Job drawing, mm, ordinate dimensions from the low corner. One solid piece. Give positions to 0.01 mm unless a question says otherwise; leave off trailing zeros. Write each loop counter-clockwise with the first axis right and the second up, starting at its lowest first coordinate (ties: lowest second). Pieces come first, ordered by that corner, then holes. Notation, with made-up numbers: M 57.25,63.25 L 115.25,63.25 A22 cw 115.25,83.25 Z; hole C 38,25 d6. An arc over 180 degrees is marked long. Use CSV: the item, a comma, the result in double quotes. Start each with the question number.
Item 1: Cut at D-D (y = 9.75). List the corners of the cut face in (x, z), then the cut area to 3 significant figures.
Item 2: Cut at C-C (x = 6.25). List the corners of the cut face in (y, z).
Item 3: Cut at A-A (x = 18.05). List the corners of the cut face in (y, z) (3 decimals).
Item 4: Pin check, flat tip, straight feed: pin 1 (2 mm diameter, centred on x = 17, z = 7.5, fed in from -Y). Stop position of the tip, or through.
Item 5: Cut at B-B (y = 2.79). List the corners of the cut face in (x, z) (3 decimals).
Item 6: Drill centre line: line 1 (Z direction, x = 7.25, y = 7.25). Where is it in solid material? Low to high. Write a range as [from, to].
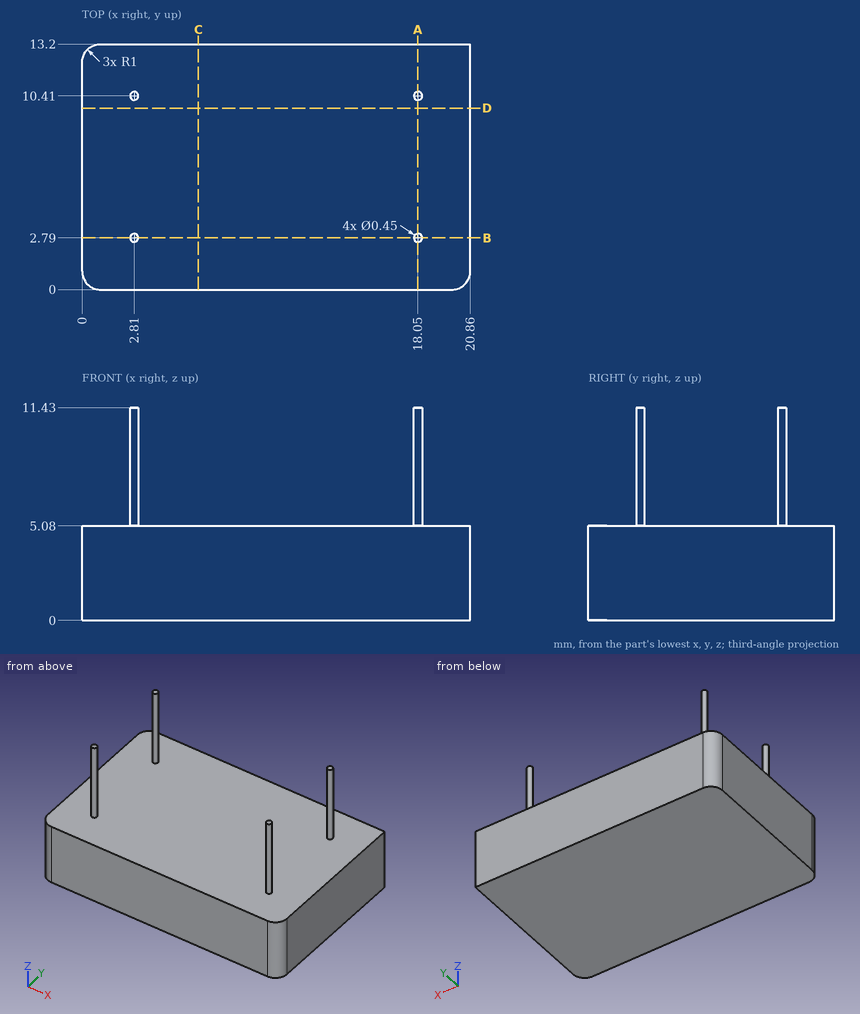
Worked answers:
1,outline,"M 0,0 L 20.86,0 L 20.86,5.08 L 0,5.08 Z"
1,area,"106 mm^2"
2,outline,"M 0,0 L 13.2,0 L 13.2,5.08 L 0,5.08 Z"
3,outline,"M 0,0 L 13.2,0 L 13.2,5.08 L 10.635,5.08 L 10.635,11.43 L 10.185,11.43 L 10.185,5.08 L 3.015,5.08 L 3.015,11.43 L 2.565,11.43 L 2.565,5.08 L 0,5.08 Z"
4,pin 1,"stops at y = 2.57"
5,outline,"M 0,0 L 20.86,0 L 20.86,5.08 L 18.275,5.08 L 18.275,11.43 L 17.825,11.43 L 17.825,5.08 L 3.035,5.08 L 3.035,11.43 L 2.585,11.43 L 2.585,5.08 L 0,5.08 Z"
6,line 1,"z = [0, 5.08]"
